Verification items for the finished model (mm, model axes). A direction names the side the tool comes from. Coordinates: 2 decimals unless noted, no trailing zeros. Loops run counter-clockwise (first coordinate to the right, second up) from the corner with the lowest first, then second, coordinate; pieces in that order, holes last. Notation, with made-up numbers: (-2, 1) -> (53, 1) arc R26 ccw to (53, 38) -> close; hole circle Ø4 at (-39, -14). An arc over 180 degrees is marked (long way). Answer as a JSON object with one key per item and string values. Group by question number.
Q1. Cross-section at A-A on y = 5. Record the boundary of the cut face in (x, z) (3 decimals), and give its area (3 significant figures).
Q2. Gauge pin test, flat ends, axial feed: pin 1 Ø11.5 at (x, z) = (-7, -8.5) entering from +Y; pin 2 Ø1.5 at (x, z) = (13, 13.5) entering from +Y (3 decimals); pin 3 Ø6 at (y, z) = (11.5, 9.5) entering from -X; pin 4 Ø2.5 at (y, z) = (5.5, 1) entering from -X (3 decimals). Record the tip position at first contact, or that the pin passes through.
Q3. Scan lines: L1, parallel to Y at x = 0, z = 0 (3 decimals); L2, parallel to Y at x = 15, z = 9 (3 decimals); L3, parallel to Y at x = 3.5, z = -2.5. Record each from-to range of solid material in increasing order.
Q4. Cross-section at D-D on z = -5. Record the boundary of the cut face in (x, y) (3 decimals).
Q5. Release check for a two-part mould opening along Y. For faces 6 (the flat face through (0, 0, 0)), 7 (the flat face through (15.875, 5, 0)), 8 (the cylindrical face through (-1.377, 3.326, -0.089)) record: released by +Y, released by -Y, zero draft, split by the parting line, or undercut.
Q6. Set-up check for faces 1 (the cylindrical face through (0.35, 22.22, 0.09)), 2 (the flat face through (-4, 15, -6.35)), 3 (the cylindrical face through (-15.12, 1.57, -11.59)), 4 (the flat face through (-4, 15, 6.35)), 5 (the flat face through (-15.875, 5, 0)): record each of +Z, -Z, +X, -X, +Y, -Y from which the full face is reachable in a straight line by a thin tool's end or side.
Q7. Cross-section at B-B on z = 0. Record the boundary of the cut face in (x, y) (3 decimals).
Q8. Cross-section at C-C on x = -14. Record the boundary of the cut face in (y, z) (3 decimals), and give its area (3 significant figures).
```python
from build123d import *

# Parameters (mm, degrees)
F1_R     = 6.35
F2_DEPTH = 6.35
F0_R     = 19.05
F0_R_2   = 9.525
F3_DEPTH = 3.175


with BuildPart() as f2:
    # F1 (on Top) → F2 (new body, symmetric)
    with BuildSketch(Plane.XY):
        with BuildLine():
            ThreePointArc((15.875, 6.35), (0, 22.225), (-15.875, 6.35))
            Line((-15.875, 6.35), (-15.875, 0))
            Line((-15.875, 0), (15.875, 0))
            Line((15.875, 0), (15.875, 6.35))
        make_face()
        with Locations((0, 9.525)):
            Circle(F1_R, mode=Mode.SUBTRACT)
    extrude(amount=F2_DEPTH, both=True)

    # F0 (on Front) → F3 (join)
    with BuildSketch(Plane.XZ):
        Circle(F0_R)
        Circle(F0_R_2, mode=Mode.SUBTRACT)
        Circle(F0_R_2)
    extrude(amount=-F3_DEPTH)


solid = f2.part
```
Computed values:
{
 "1": {"outline": "(-15.875, -6.35) -> (-4.455, -6.35) -> (-4.455, 6.35) -> (-15.875, 6.35) -> close; (4.455, -6.35) -> (15.875, -6.35) -> (15.875, 6.35) -> (4.455, 6.35) -> close", "area": "290 mm²"},
 "2": {"pin 1": "stops at y = 22.14", "pin 2": "stops at y = 3.175", "pin 3": "passes through", "pin 4": "stops at x = -15.875"},
 "3": {"L1": "y = 0 to 3.175, 15.875 to 22.225", "L2": "y = 0 to 3.175", "L3": "y = 0 to 4.23, 14.82 to 21.83"},
 "4": {"outline": "(-18.382, 0) -> (18.382, 0) -> (18.382, 3.175) -> (15.875, 3.175) -> (15.875, 6.35) arc R15.875 ccw to (-15.875, 6.35) -> (-15.875, 3.175) -> (-18.382, 3.175) -> close; hole circle Ø12.7 at (0, 9.525)"},
 "5": {"face 6": "released by -Y", "face 7": "zero draft", "face 8": "undercut"},
 "6": {"face 1": "+Z, -Z, +Y", "face 2": "-Z, +X, -X, +Y", "face 3": "+Y, -Y", "face 4": "+Z, +X, -X, +Y", "face 5": "+Z, -Z, -X, +Y"},
 "7": {"outline": "(-19.05, 0) -> (19.05, 0) -> (19.05, 3.175) -> (15.875, 3.175) -> (15.875, 6.35) arc R15.875 ccw to (-15.875, 6.35) -> (-15.875, 3.175) -> (-19.05, 3.175) -> close; hole circle Ø12.7 at (0, 9.525)"},
 "8": {"outline": "(0, -12.919) -> (3.175, -12.919) -> (3.175, -6.35) -> (13.834, -6.35) -> (13.834, 6.35) -> (3.175, 6.35) -> (3.175, 12.919) -> (0, 12.919) -> close", "area": "217 mm²"}
}
